Geometry: final body of the model. Coordinates: model frame, mm. A direction names the side the tool comes from. Coordinates: 2 decimals unless noted, no trailing zeros. Write each loop counter-clockwise with the first axis right and the second up, starting at its lowest first coordinate (ties: lowest second). Pieces come first, ordered by that corner, then holes. Notation, with made-up numbers: (85.5, -26.5) -> (120.5, -26.5) arc R13 cw to (120.5, -3.5) -> close; hole circle Ø6 at (-10, 2.25). An arc over 180 degrees is marked (long way). Answer as a JSON object with one key per item and string values. Group by question number.
```python
from build123d import *

# Parameters (mm, degrees)
SKETCH1_W                                        = 38.1
SKETCH1_H                                        = 50
BOSS_EXTRUDE1_DEPTH                              = 69.85
CBORE_FOR_1_2_SOCKET_HEAD_CAP_SCREW1_D           = 13.89126
CBORE_FOR_1_2_SOCKET_HEAD_CAP_SCREW1_CBORE_D     = 20.6375
CBORE_FOR_1_2_SOCKET_HEAD_CAP_SCREW1_CBORE_DEPTH = 27.94
CUT_EXTRUDE1_DEPTH                               = 6
CUT_EXTRUDE2_DEPTH                               = 4
FILLET1_R                                        = 0.254


with BuildPart() as part:
    # Sketch1 → Boss-Extrude1 (new body, symmetric)
    with BuildSketch(Plane(origin=(0, 0, 0), x_dir=(0, 0, -1), z_dir=(1, 0, 0))):
        Rectangle(SKETCH1_W, SKETCH1_H)
    extrude(amount=BOSS_EXTRUDE1_DEPTH, both=True)

    # CBORE for 1/2 Socket Head Cap Screw1 (through all)
    with Locations(Plane.XY.offset(19.05)):
        with Locations((-49.2125, -1.124), (49.2125, -1.124)):
            CounterBoreHole(CBORE_FOR_1_2_SOCKET_HEAD_CAP_SCREW1_D / 2, CBORE_FOR_1_2_SOCKET_HEAD_CAP_SCREW1_CBORE_D / 2, CBORE_FOR_1_2_SOCKET_HEAD_CAP_SCREW1_CBORE_DEPTH)

    # Sketch5 → Cut-Extrude1 (cut)
    with BuildSketch(Plane(origin=(0, 25, 0), x_dir=(1, 0, 0), z_dir=(0, 1, 0))):
        with BuildLine():
            Line((-36.1, -19.05), (-30.1, -19.05))
            ThreePointArc((-30.1, -19.05), (-33.1, -16.05), (-36.1, -19.05))
        make_face()
        with BuildLine():
            Line((36.1, -19.05), (30.1, -19.05))
            ThreePointArc((30.1, -19.05), (33.1, -16.05), (36.1, -19.05))
        make_face()
    extrude(amount=-CUT_EXTRUDE1_DEPTH, mode=Mode.SUBTRACT)

    # Sketch7 → Cut-Extrude2 (cut)
    with BuildSketch(Plane(origin=(0, 25, 0), x_dir=(1, 0, 0), z_dir=(0, 1, 0))):
        with BuildLine():
            Line((45.85, -14.05), (45.85, -19.05))
            Line((45.85, -19.05), (65.85, -19.05))
            Line((65.85, -19.05), (65.85, -14.05))
            ThreePointArc((65.85, -14.05), (63.85, -12.05), (61.85, -14.05))
            Line((61.85, -14.05), (49.85, -14.05))
            ThreePointArc((49.85, -14.05), (47.85, -12.05), (45.85, -14.05))
        make_face()
        with BuildLine():
            Line((-61.85, -14.05), (-49.85, -14.05))
            ThreePointArc((-49.85, -14.05), (-47.85, -12.05), (-45.85, -14.05))
            Line((-45.85, -14.05), (-45.85, -19.05))
            Line((-45.85, -19.05), (-65.85, -19.05))
            Line((-65.85, -19.05), (-65.85, -14.05))
            ThreePointArc((-65.85, -14.05), (-63.85, -12.05), (-61.85, -14.05))
        make_face()
    extrude(amount=-CUT_EXTRUDE2_DEPTH, mode=Mode.SUBTRACT)

    # Fillet1
    fillet1_edges = [part.edges().sort_by_distance(p)[0] for p in [
        (49.85, 23, 14.05),
        (61.85, 23, 14.05),
        (-61.85, 23, 14.05),
        (-49.85, 23, 14.05),
    ]]
    fillet(fillet1_edges, radius=FILLET1_R)


solid = part.part
```
Item 1: Section C-C on z = -7. Output: boundary loops of the cut face in (x, y).
Item 2: Section A-A on x = 47.85. Output: boundary loops of the cut face in (y, z).
Item 3: Mould query, pull axis Y, two halves, no side actions, for faces 1 (the flat face through (-33, 19, 18)), 2 (the cylindrical face through (-39.37, 1.98, 5.28)), 3 (the flat face through (1, 0, -19.05)). Classes: +Y half, -Y half, draft (parallel to the pull), parting line (faces both ways), or undercut.
Item 4: Contact query for flat-ended pins moving along their axis: pin 1 (18 mm diameter, centred on x = -49.21, y = -1.12, fed in from +Z); pin 2 (1.2 mm diameter, centred on x = -56, y = 23.5, fed in from +Z). Output: stop coordinate, or through.
Item 5: Set-up query: faces 4 (the flat face through (-65.85, 23, 17)), 5 (the flat face through (-42, -3, -8.89)), 6 (the flat face through (-69.85, 0, 0)). Return all of +Z, -Z, +X, -X, +Y, -Y with unobstructed straight access to the full face (end or side cutting, diameter ignored); none if empty.
Item 6: Section B-B on y = -5. Output: boundary loops of the cut face in (x, z).
Item 7: Ray query, L1, parallel to X at y = 2.5, z = -9.5; L2, parallel to X at y = 1.5, z = 15; L3, parallel to Y at x = -45, z = 5.5. Return the intervals inside material, ascending. Write a range as [from, to].
Item 8: Section D-D on z = -13.5. Output: boundary loops of the cut face in (x, y).
Answer sheet:
{
 "1": {"outline": "(-69.85, -25) -> (69.85, -25) -> (69.85, 25) -> (-69.85, 25) -> close; hole circle Ø20.64 at (-49.21, -1.12); hole circle Ø20.64 at (49.21, -1.12)"},
 "2": {"outline": "(-25, -19.05) -> (-7.93, -19.05) -> (-7.93, -8.89) -> (-11.35, -8.89) -> (-11.35, 19.05) -> (-25, 19.05) -> close; (5.69, -19.05) -> (25, -19.05) -> (25, 12.05) -> (21, 12.05) -> (21, 19.05) -> (9.1, 19.05) -> (9.1, -8.89) -> (5.69, -8.89) -> close"},
 "3": {"face 1": "+Y half", "face 2": "undercut", "face 3": "draft"},
 "4": {"pin 1": "stops at z = -8.89", "pin 2": "stops at z = 14.05"},
 "5": {"face 4": "+Z, +Y", "face 5": "+Z", "face 6": "+Z, -Z, -X, +Y, -Y"},
 "6": {"outline": "(-69.85, -19.05) -> (-54.98, -19.05) -> (-54.98, -8.89) -> (-58.78, -8.89) -> (-58.78, 19.05) -> (-69.85, 19.05) -> close; (-43.45, -19.05) -> (43.45, -19.05) -> (43.45, -8.89) -> (39.65, -8.89) -> (39.65, 19.05) -> (-39.65, 19.05) -> (-39.65, -8.89) -> (-43.45, -8.89) -> close; (54.98, -19.05) -> (69.85, -19.05) -> (69.85, 19.05) -> (58.78, 19.05) -> (58.78, -8.89) -> (54.98, -8.89) -> close"},
 "7": {"L1": "x = [-69.85, -55.14], [-43.29, 43.29], [55.14, 69.85]", "L2": "x = [-69.85, -59.19], [-39.23, 39.23], [59.19, 69.85]", "L3": "y = [-25, -10.54], [8.3, 25]"},
 "8": {"outline": "(-69.85, -25) -> (69.85, -25) -> (69.85, 25) -> (-69.85, 25) -> close; hole circle Ø13.89 at (-49.21, -1.12); hole circle Ø13.89 at (49.21, -1.12)"}
}
